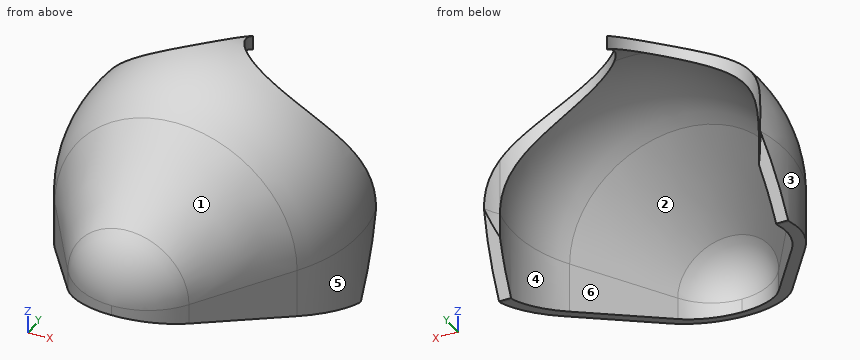
from build123d import *

# Parameters (mm, degrees)
F1_ANGLE = 180
F2_DEPTH = 76.201
F3_DEPTH = 38.1
F5_DEPTH = 127


# Not quite as in the source:
# - a feature names something its author has since deleted; it is built from what else it names


with BuildPart() as f1:
    # F0 (on Top) → F1 (revolve)
    with BuildSketch(Plane.XY):
        with BuildLine():
            ThreePointArc((0, 69.85), (43.8400236241, 54.3789925306), (68.2598802346, 14.819286432))
            ThreePointArc((68.2598802346, 14.819286432), (70.7649049458, 18.4884221725), (72.8257812379, 22.4242187621))
            ThreePointArc((72.8257812379, 22.4242187621), (45.2643045364, 61.299125074), (0, 76.2))
            Line((0, 76.2), (0, 69.85))
        make_face()
        with BuildLine():
            Line((58.5441073038, -38.1), (26.6109578654, -87.1681818182))
            ThreePointArc((26.6109578654, -87.1681818182), (15.1362186043, -97.7598080675), (0, -101.6))
            Line((0, -101.6), (0, -107.95))
            ThreePointArc((0, -107.95), (18.1634623251, -103.341769681), (31.9331494384, -90.6318181818))
            Line((31.9331494384, -90.6318181818), (63.8662988769, -41.5636363636))
            ThreePointArc((63.8662988769, -41.5636363636), (75.4638495733, -10.5663336866), (72.8257812379, 22.4242187621))
            ThreePointArc((72.8257812379, 22.4242187621), (70.7649049458, 18.4884221725), (68.2598802346, 14.819286432))
            ThreePointArc((68.2598802346, 14.819286432), (68.7017141928, -12.6133646173), (58.5441073038, -38.1))
        make_face()
    revolve(axis=Axis((0, -12.7, 0), (0, -1, 0)), revolution_arc=F1_ANGLE)

    # F0 (on Top) → F2 (cut, through all)
    with BuildSketch(Plane.XY):
        with BuildLine():
            ThreePointArc((0, 38.1), (25.8012487817, 2.0396239832), (68.2598802346, 14.819286432))
            ThreePointArc((68.2598802346, 14.819286432), (43.8400236241, 54.3789925306), (0, 69.85))
            Line((0, 69.85), (0, 76.2))
            ThreePointArc((0, 76.2), (45.2643045364, 61.299125074), (72.8257812379, 22.4242187621))
            ThreePointArc((72.8257812379, 22.4242187621), (70.1066966834, 58.7683663461), (38.1, 76.2))
            ThreePointArc((38.1, 76.2), (0, 114.3), (-38.1, 76.2))
            ThreePointArc((-38.1, 76.2), (-65.0407683632, 11.1592316368), (0, 38.1))
        make_face()
        with BuildLine():
            ThreePointArc((0, 69.85), (43.8400236241, 54.3789925306), (68.2598802346, 14.819286432))
            ThreePointArc((68.2598802346, 14.819286432), (70.7649049458, 18.4884221725), (72.8257812379, 22.4242187621))
            ThreePointArc((72.8257812379, 22.4242187621), (45.2643045364, 61.299125074), (0, 76.2))
            Line((0, 76.2), (0, 69.85))
        make_face()
    extrude(amount=F2_DEPTH, mode=Mode.SUBTRACT)

    # F3 (add): a face of the model
    f3_faces = [f1.faces().sort_by_distance(p)[0] for p in [
        (72.4843753918, 17.4560748099, 0),
    ]]
    extrude(f3_faces, amount=F3_DEPTH)

    # F4 (on Right) → F5 (cut, symmetric)
    with BuildSketch(Plane.YZ):
        Polygon((22.4127881229, 0), (0, -38.3907258511), (-2.2853469058, -42.3052824003), (29.7282127851, -42.3052824003), (29.7282127851, 12.5305455596), align=None)
        Polygon((-125.4685521126, -38.3907258511), (0, -38.3907258511), (-125.4685521126, 0), align=None)
    extrude(amount=F5_DEPTH, both=True, mode=Mode.SUBTRACT)


solid = f1.part
Work out the finished part from the listing and answer in its coordinate system (mm). Face numbers are marked on the shaded views. A direction names the side the tool comes from. Give positions to 0.01 mm unless a question says otherwise; leave off trailing zeros. Write each loop counter-clockwise with the first axis right and the second up, starting at its lowest first coordinate (ties: lowest second). Pieces come first, ordered by that corner, then holes. Notation, with made-up numbers: M 64,-31.5 L 97,-31.5 A15 ccw 97,-27.5 Z; hole C -24,29 d2. An arc over 180 degrees is marked long. Answer as CSV lines item,"result".
Q1. A tool of negligible diameter and unlimited length cuts with its end or side. For the marked faces 5 and 6, from which of +Z, -Z, +X, -X, +Y, -Y can it reach the whole face along a straight path? Write none if from no direction.
A:
face 5,"+Z, -Z, +X"
face 6,"-Z, +Y"
Q2. Find the intervals of material crossed by probe 1 along X at (y, z) = (-76, 30); probe 2 along X at (y, z) = (-43, 11); probe 3 along Y at (x, z) = (-30, 45.5), in increasing order. Write a range as [from, to].
A:
probe 1,"x = [-28.61, -15.74], [15.74, 28.61]"
probe 2,"x = [-61.96, -54.25], [54.25, 61.96]"
probe 3,"y = [-55.96, -44.31]"
Q3. The mould has two halves that part along Y. Classify the marked faces 1, 2, 3 and 4: +Y half, -Y half, draft (parallel to the pull), parting line (faces both ways), or undercut.
A:
face 1,"-Y half"
face 2,"+Y half"
face 3,"parting line"
face 4,"undercut"
Q4. A cutting plane is placed at A-A on y = 20. Write down the section's boundary in (x, z).
A:
outline,"M -73.53,-4.13 L -71.63,-4.13 L -71.63,16.62 A73.53 ccw -73.53,0 Z; M -4.57,66.77 A66.93 cw 4.57,66.77 L 4.57,73.39 A73.53 ccw -4.57,73.39 Z; M 71.63,-4.13 L 73.53,-4.13 L 73.53,0 A73.53 ccw 71.63,16.62 Z"
Q5. Given P1, Ø6, axis at x = 18.5, z = 1.5, coming from the -Y side; P2, Ø10, axis at x = 48.5, z = 50.5, coming from the +Y side; P3, Ø5, axis at x = -12.5, z = 59.5, coming from the -Y side, each flat-ended and moving along its own axis, determine where each tip first touches the part or whether it passes through.
A:
P1,"stops at y = -104.63"
P2,"stops at y = 3.25"
P3,"stops at y = -50.12"
Q6. A cutting plane is placed at B-B on y = -17. Write down the section's boundary in (x, z), plus the area to 3 significant figures.
A:
outline,"M -74.28,-33.19 L -67.75,-33.19 L -67.75,0 A67.75 cw 67.75,0 L 67.75,-33.19 L 74.28,-33.19 L 74.28,0 A74.28 ccw -74.28,0 Z"
area,"1,890 mm²"
Q7. A cutting plane is placed at D-D on y = -79.5. Write down the section's boundary in (x, z).
A:
outline,"M -39.18,-14.07 L -31.6,-14.07 L -31.6,0 A31.6 cw 31.6,0 L 31.6,-14.07 L 39.18,-14.07 L 39.18,0 A39.18 ccw -39.18,0 Z"
Q8. A cutting plane is placed at C-C on x = -66. Write down the section's boundary in (y, z).
A:
outline,"M -38.08,-26.74 L -22.87,-31.39 L -22.87,0 A22.87 cw 12.15,19.37 L 12.15,36.09 A38.08 ccw -38.08,0 Z"
